Autodesk Inventor part; units mm, degrees
ref_plane "YZ Plane" through (0, 0, 0) normal (1, 0, 0) x (0, 1, 0)
ref_plane "XZ Plane" through (0, 0, 0) normal (0, 1, 0) x (-1, 0, 0)
ref_plane "XY Plane" through (0, 0, 0) normal (0, 0, 1) x (1, 0, 0)
sketch "Sketch1" plane through (0, 0, 0) normal (1, 0, 0) x (0, 1, 0)
  line L0 (-76.2, 25.8729) -> (-203.2, 25.8729)
  line L1 (-203.2, 25.8729) -> (-203.2, -355.1271)
  line L2 (-203.2, -355.1271) -> (-76.2, -355.1271)
  line L3 (-76.2, -355.1271) -> (-76.2, 25.8729)
  point P0 (0, 0)
  dimension "d0" = 127
  dimension "d1" = 381
extrude "Extrusion1" add sketch "Sketch1" along normal blind 7.62
sketch "Sketch2" plane through (7.62, 0, 0) normal (1, 0, 0) x (0, 0, -1)
  circle A0 centre (0, -187.325) radius 11.9854
  circle A1 centre (334.9625, -187.325) radius 11.557
  point P0 (0, 0)
  dimension "d5" = 23.114
extrude "Extrusion2" add sketch "Sketch2" along normal blind 114.3
sketch "Sketch3" plane through (7.62, 0, 0) normal (1, 0, 0) x (0, 0, -1)
  circle A0 centre (0, -93.6625) radius 11.557
  circle A1 centre (334.9625, -93.6625) radius 11.557
  point P0 (0, 0)
  dimension "d8" = 23.114
  dimension "d9" = 23.114
extrude "Extrusion3" add sketch "Sketch3" along normal blind 114.3
sketch "Sketch4" plane through (0, 0, 0) normal (-1, 0, 0) x (0, 0, 1)
  line L0 (25.8729, -76.2) -> (25.8729, -203.2)
  line L1 (-355.1271, -203.2) -> (-355.1271, -76.2)
  line L2 (25.8729, -203.2) -> (-355.1271, -203.2)
  line L3 (-355.1271, -203.2) -> (-355.1271, -196.85)
  line L4 (-355.1271, -196.85) -> (25.8729, -196.85)
  line L5 (25.8729, -196.85) -> (25.8729, -203.2)
  line L6 (-355.1271, -76.2) -> (25.8729, -76.2)
  line L7 (-355.1271, -196.85) -> (-347.1769, -196.85)
  line L8 (-347.1769, -196.85) -> (-347.1769, -76.2)
  line L9 (-347.1769, -76.2) -> (-355.1271, -76.2)
  line L10 (-355.1271, -76.2) -> (-355.1271, -196.85)
  line L11 (25.8729, -84.1375) -> (-355.1271, -84.1375)
  line L12 (-355.1271, -84.1375) -> (-355.1271, -76.2)
  line L13 (-355.1271, -76.2) -> (25.8729, -76.2)
  line L14 (25.8729, -76.2) -> (25.8729, -84.1375)
  point P0 (0, 0)
  point P1 (25.8729, -196.85)
  point P2 (-347.1769, -84.1375)
  dimension "d12" = 7.9502
extrude "Extrusion4" add sketch "Sketch4" along normal blind 17.78 contours L0 L11 L8 L6 | L8 L11 L1 L6 | L0 L2 L1 L4 | L8 L4 L1 L11
properties part number "TABLE FOR VERTI" material "Wood (Maple)"
The listing builds one solid part. Answer for the finished solid, in the listing's coordinates (mm). A direction names the side the tool comes from. Coordinates: 2 decimals unless noted, no trailing zeros. Write each loop counter-clockwise with the first axis right and the second up, starting at its lowest first coordinate (ties: lowest second). Pieces come first, ordered by that corner, then holes. Notation, with made-up numbers: M 34,23.5 L 50,23.5 A21 cw 50,35.5 Z; hole C 51,84.5 d9. An arc over 180 degrees is marked long. Use a Markdown table: item, result. Add a question column.
1. Section C-C (x = 48.5) is taken. Give the vertices of the cut face in (y, z) (1 decimal), plus the area to 3 significant figures.
2. Section D-D (z = 0) is taken. Give the vertices of the cut face in (x, y), plus the area to 3 significant figures.
3. Given P1, Ø8, axis at y = -122, z = -23.5, coming from the -X side; P2, Ø12, axis at x = 41, y = -110, coming from the +Z side; P3, Ø6, axis at y = -158.5, z = -182, coming from the +X side, each flat-ended and moving along its own axis, determine where each tip first touches the part or whether it passes through.
4. For a pull along Y with two mould halves and no side action, classify faces 1 (the flat face through (-9, -141, -347.177)), 2 (the flat face through (-5, -76.2, -167)), 3 (the flat face through (121.92, -94, 0)), 4 (the flat face through (-5, -203.2, -162)) as +Y half, -Y half, draft (parallel to the pull), parting line (faces both ways), or undercut.
5. Which of the six approach directions +Z, -Z, +X, -X, +Y, -Y give full straight-line access (tool end or side, diameter ignored) to faces 5 (the flat face through (-5, -141, -355.127)), 6 (the cylindrical face through (63.97, -190.796, -345.986)), 7 (the flat face through (-9, -84.138, -158))?
6. Straight lines are drawn through the part: line 1 along X through (y, z) = (-125, -87.5); line 2 along Z through (x, y) = (-3.5, -120); line 3 along Y through (x, z) = (48, -335.5). For each, find the intervals that lie inside material, in ascending order. Write a range as [from, to].
7. Section B-B (y = -121.5) is taken. Give the vertices of the cut face in (x, z).
8. Section A-A (z = -76.5) is taken. Give the vertices of the cut face in (x, y), plus the area to 3 significant figures.
Data:
| question | item | result |
|---|---|---|
| 1 | outline | C -187.3,0 d24; C -187.3,-335 d23.1; C -93.7,-335 d23.1; C -93.7,0 d23.1 |
| 1 | area | 1,710 mm2 |
| 2 | outline | M -17.78,-203.2 L 7.62,-203.2 L 7.62,-199.31 L 121.92,-199.31 L 121.92,-175.34 L 7.62,-175.34 L 7.62,-105.22 L 121.92,-105.22 L 121.92,-82.11 L 7.62,-82.11 L 7.62,-76.2 L -17.78,-76.2 L -17.78,-84.14 L 0,-84.14 L 0,-196.85 L -17.78,-196.85 Z |
| 2 | area | 6,600 mm2 |
| 3 | P1 | stops at x = 0 |
| 3 | P2 | stops at z = 5.17 |
| 3 | P3 | stops at x = 7.62 |
| 4 | face 1 | undercut |
| 4 | face 2 | +Y half |
| 4 | face 3 | draft |
| 4 | face 4 | -Y half |
| 5 | face 5 | -Z, +X, -X, +Y, -Y |
| 5 | face 6 | +X |
| 5 | face 7 | +Z, -X |
| 6 | line 1 | x = [0, 7.62] |
| 6 | line 2 | z = [-355.13, -347.18] |
| 6 | line 3 | y = [-198.87, -175.78], [-105.21, -82.12] |
| 7 | outline | M -17.78,-355.13 L 7.62,-355.13 L 7.62,25.87 L 0,25.87 L 0,-347.18 L -17.78,-347.18 Z |
| 8 | outline | M -17.78,-203.2 L 7.62,-203.2 L 7.62,-76.2 L -17.78,-76.2 L -17.78,-84.14 L 0,-84.14 L 0,-196.85 L -17.78,-196.85 Z |
| 8 | area | 1,220 mm2 |
